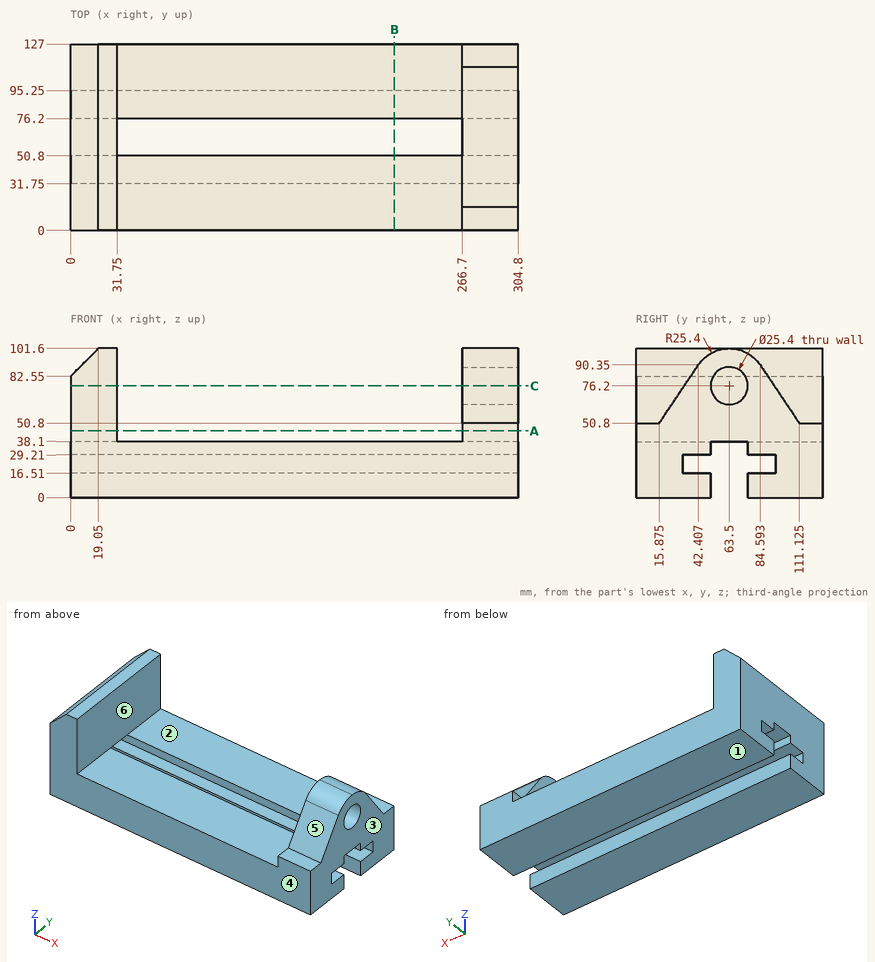
Design review of the part shown in the three views and the two pictorial views. Dimensions are in mm from the part's minimum x, y and z. A direction names the side the tool comes from. Give positions to 0.01 mm unless a question says otherwise; leave off trailing zeros. Loops run counter-clockwise (first coordinate to the right, second up) from the corner with the lowest first, then second, coordinate; pieces in that order, holes last. Notation, with made-up numbers: M -40,11.25 L 18,11.25 A18 ccw 18,29.25 Z; hole C -11.75,77.5 d10. An arc over 180 degrees is marked long. Write item = value, one per line.
Q1. To check wall thickness, follow line 1 (Y direction, x = 182, z = 24.5); line 2 (X direction, y = 29, z = 43); line 3 (Z direction, x = 284, y = 63.5). State the ranges of each line that lie inside material, in increasing order. Write a range as [from, to].
Output values:
line_1 = [0, 31.75], [95.25, 127]
line_2 = [0, 31.75], [266.7, 304.8]
line_3 = [38.1, 63.5], [88.9, 101.6]
Q2. We need section A-A (z = 45.5). Give the boundary of the cut face in (x, y), plus the area to 3 significant figures.
Output values:
outline = M 0,0 L 31.75,0 L 31.75,127 L 0,127 Z; M 266.7,0 L 304.8,0 L 304.8,127 L 266.7,127 Z
area = 8,870 mm^2
Q3. Draft analysis for pull direction X (two halves, no side actions). For the marked faces 1, 2 and 3, state which applies: +X half, -X half, draft (parallel to the pull), parting line (faces both ways), or undercut.
Output values:
face_1 = draft
face_2 = undercut
face_3 = +X half
Q4. We need section B-B (x = 220.5). Give the boundary of the cut face in (y, z), plus the area to 3 significant figures.
Output values:
outline = M 0,0 L 50.8,0 L 50.8,16.51 L 31.75,16.51 L 31.75,29.21 L 50.8,29.21 L 50.8,38.1 L 0,38.1 Z; M 76.2,0 L 127,0 L 127,38.1 L 76.2,38.1 L 76.2,29.21 L 95.25,29.21 L 95.25,16.51 L 76.2,16.51 Z
area = 3,390 mm^2
Q5. For the marked faces 4, 5 and 6, list the 3-axis set-ups (+Z, -Z, +X, -X, +Y, -Y) from which the entire face can be reached by the end or side of a thin tool; tool diameter is ignored.
Output values:
face_4 = +Z, -Z, +X, -X, -Y
face_5 = +Z, +X, -Y
face_6 = +Z, +Y, -Y
Q6. Insertion check: pin 1 (2 mm diameter, centred on x = 115.5, y = 114, fed in from +Z); pin 2 (12.5 mm diameter, centred on x = 287, y = 6, fed in from +Z). Each pin has a flat end and moves straight along its axis. Give the tip position at first contact, or say it passes through.
Output values:
pin_1 = 38.1
pin_2 = 50.8
Q7. We need section C-C (z = 76.2). Count the separate pieces of the cut face and the enclosed holes in it.
Output values:
separate_pieces = 3
enclosed_holes = 0
